The drawing under review shows one solid part. Ordinate dimensions are in mm from its lowest x, y, z. A direction names the side the tool comes from. Round coordinates to 2 decimals unless told otherwise and drop trailing zeros. Write each loop counter-clockwise with the first axis right and the second up, starting at its lowest first coordinate (ties: lowest second). Pieces come first, ordered by that corner, then holes. Notation, with made-up numbers: (45.5, 0.5) - (102.5, 0.5) arc R22 ccw to (102.5, 35.5) - close; hole circle Ø2 at (37, -40). An arc over 180 degrees is marked (long way). One line per question, with ' | ' between items. Start each with the question number.
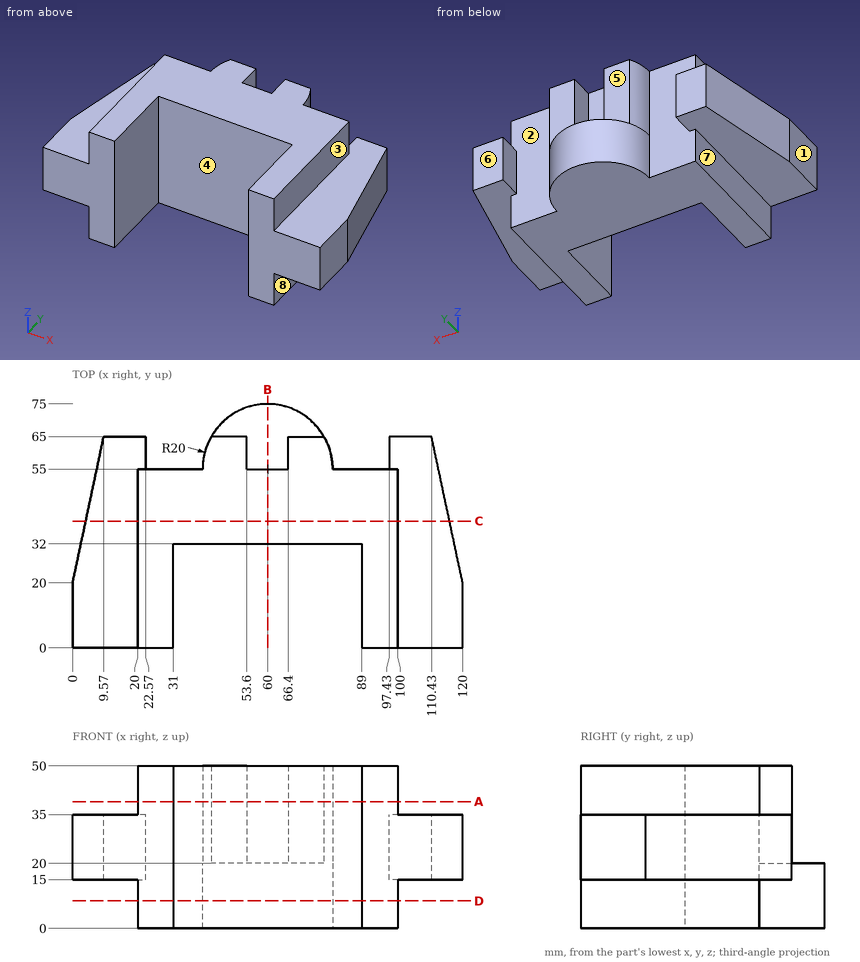
1. Add section A-A, the plane z = 39. Write out the cut boundary in (x, y), then the cut area to 3 significant figures.
2. The part is to be moulded in two halves that separate along X. For the marked faces 1, 2 and 3, say which applies: pulls with the +X half, pulls with the -X half, needs draft (parallel to the pull), parting line crosses it, or undercut.
3. Machinability: for the marked faces 4, 5, 6, 7 and 8, which of the approach directions +Z, -Z, +X, -X, +Y, -Y give a long, thin tool a straight path to every point of the face, cutting with its end or side? Answer none if there is none.
4. Clearance check with flat-ended pins moving along their axes: P1, Ø8, axis at x = 70.5, z = 22.5, coming from the -Y side; P2, Ø16, axis at x = 90.5, z = 28.5, coming from the +Y side; P3, Ø4.5, axis at y = 32.5, z = 42, coming from the -X side. State where each tip first meets the part, or that it passes through.
5. Wall thickness on line 1 along X through (y, z) = (28.5, 7); line 2 along Z through (x, y) = (59, 63.5); line 3 along X through (y, z) = (61.5, 22): over which ranges is each line inside the solid? List them lowest first. Write a range as [from, to].
6. Add section B-B, the plane x = 60. Write out the cut boundary in (y, z), then the cut area to 3 significant figures.
7. Add section D-D, the plane z = 8.5. Write out the cut boundary in (x, y).
8. Add section C-C, the plane y = 39. Write out the cut boundary in (x, z), then the cut area to 3 significant figures.
Geometry check:
1) outline: (20, 0) - (31, 0) - (31, 32) - (89, 32) - (89, 0) - (100, 0) - (100, 55) - (80, 55) arc R20 ccw to (77.32, 65) - (66.4, 65) - (66.4, 55) - (53.6, 55) - (53.6, 65) - (42.68, 65) arc R20 ccw to (40, 55) - (20, 55) - close | area: 2,800 mm2
2) face 1: pulls with the -X half | face 2: undercut | face 3: pulls with the +X half
3) face 4: +Z, -Z, -Y | face 5: +Z, +X, -X, +Y | face 6: +Z, -Z, +X, +Y | face 7: -Z, -X, +Y, -Y | face 8: -Z, +X, +Y, -Y
4) P1: stops at y = 32 | P2: stops at y = 65 | P3: stops at x = 20
5) line 1: x = [20, 31], [89, 100] | line 2: z = [0, 20] | line 3: x = [8.83, 22.57], [41.09, 53.6], [66.4, 78.91], [97.43, 111.17]
6) outline: (32, 0) - (75, 0) - (75, 20) - (55, 20) - (55, 50) - (32, 50) - close | area: 1,550 mm2
7) outline: (20, 0) - (31, 0) - (31, 32) - (89, 32) - (89, 0) - (100, 0) - (100, 55) - (80, 55) arc R20 ccw to (40, 55) - (20, 55) - close
8) outline: (4.04, 15) - (20, 15) - (20, 0) - (100, 0) - (100, 15) - (115.96, 15) - (115.96, 35) - (100, 35) - (100, 50) - (20, 50) - (20, 35) - (4.04, 35) - close | area: 4,640 mm2
